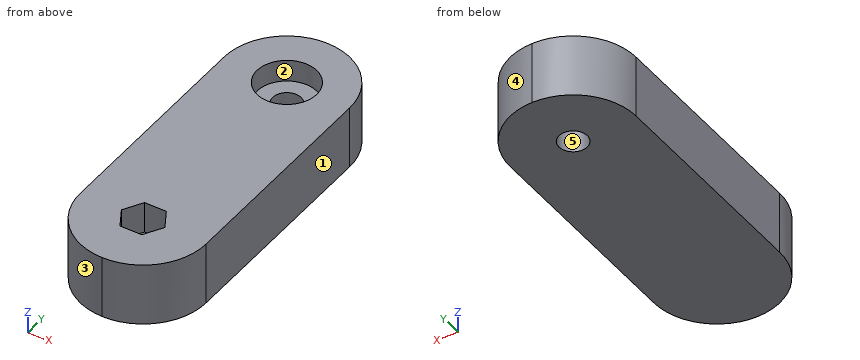
Solid Edge part; units mm, degrees
sketch "Sketch1" plane through (0, 0, 0) normal (0, -1, 0) x (1, 0, 0)
  line L0 (20, 10) -> (-20, 10)
  line L1 (-20, 10) -> (-20, -10)
  line L2 (-20, -10) -> (20, -10)
  line L3 (20, -10) -> (20, 10)
extrude "Protrusion1" add sketch "Sketch1" against normal blind 110
fillet "Redondeo_2" radius 20 4 edges at (20, 0, 0) (-20, 0, 0) (20, 110, 0) (-20, 110, 0)
sketch "Sketch2" plane through (0, 95, 10) normal (0, 0, 1) x (0, 1, 0)
  line L0 (-75, -6.9282) -> (-69, -3.4641)
  line L1 (-69, -3.4641) -> (-69, 3.4641)
  line L2 (-69, 3.4641) -> (-75, 6.9282)
  line L3 (-75, 6.9282) -> (-81, 3.4641)
  line L4 (-81, 3.4641) -> (-81, -3.4641)
  line L5 (-81, -3.4641) -> (-75, -6.9282)
extrude "VaciadoExtruido_16" cut sketch "Sketch2" against normal blind 10
sketch "Sketch3" plane through (0, 95, 10) normal (0, 0, 1) x (0, 1, 0)
  circle A0 centre (-5, 0) radius 4.5
extrude "VaciadoExtruido_17" cut sketch "Sketch3" against normal blind 52.6544
sketch "Sketch4" plane through (0, 95, 10) normal (0, 0, 1) x (0, 1, 0)
  circle A0 centre (-5, 0) radius 9.5
extrude "VaciadoExtruido_18" cut sketch "Sketch4" against normal blind 7
Geometry: final body of the model. Coordinates: model frame, mm. Face numbers are marked on the shaded views. A direction names the side the tool comes from. Round coordinates to 2 decimals unless told otherwise and drop trailing zeros. Loops run counter-clockwise (first coordinate to the right, second up) from the corner with the lowest first, then second, coordinate; pieces in that order, holes last. Notation, with made-up numbers: (64, -26) -> (96, -26) arc R12 ccw to (96, -20) -> close; hole circle Ø7 at (-16, 88). An arc over 180 degrees is marked (long way). Use one line per item in the form item = value.
Item 1: Draft query along Y for the marked faces 3, 4 and 5. Return one class per face: released by +Y, released by -Y, zero draft, split by the parting line, or undercut.
Evaluation:
face_3 = released by -Y
face_4 = released by +Y
face_5 = undercut
Item 2: Cut plane D-D on x = -16. Output: boundary loops of the cut face in (y, z), then the cut area to 3 significant figures.
Evaluation:
outline = (8, -10) -> (102, -10) -> (102, 10) -> (8, 10) -> close
area = 1,880 mm2
Item 3: Cut plane A-A on z = 1. Give the number of separate pieces and of enclosed holes in the cut face, then the cut area to 3 significant figures.
Evaluation:
separate_pieces = 1
enclosed_holes = 2
area = 3,870 mm2
Item 4: Material intervals for probe 1 along Y at (x, z) = (0, 6.5); probe 2 along X at (y, z) = (90, -7); probe 3 along X at (y, z) = (90, 7), sorted ascending.
Evaluation:
probe_1 = 0 to 14, 26 to 80.5, 99.5 to 110
probe_2 = -20 to -4.5, 4.5 to 20
probe_3 = -20 to -9.5, 9.5 to 20
Item 5: Access query for the marked faces 1 and 2. Directions: +Z, -Z, +X, -X, +Y, -Y. A direction counts if a zero-diameter tool reaches every point of the face in a straight line with its end or side. Return the directions, or none.
Evaluation:
face_1 = +Z, -Z, +X, +Y, -Y
face_2 = +Z
Item 6: Contact query for flat-ended pins moving along their axis: pin 1 Ø11.5 at (x, y) = (0, 90) entering from -Z; pin 2 Ø8 at (x, z) = (16, 6.5) entering from -Y; pin 3 Ø1 at (x, z) = (4.5, 4.5) entering from +Y; pin 4 Ø8 at (x, y) = (0, 90) entering from +Z. Output: stop coordinate, or through.
Evaluation:
pin_1 = -10
pin_2 = 4
pin_3 = 109.6
pin_4 = through
Item 7: Cut plane C-C on x = -10.5. Output: boundary loops of the cut face in (y, z).
Evaluation:
outline = (2.98, -10) -> (107.02, -10) -> (107.02, 10) -> (2.98, 10) -> close
